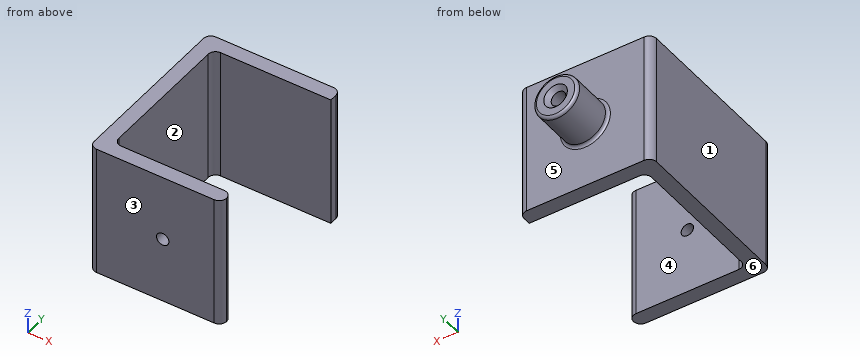
```python
from build123d import *

# Parameters (mm, degrees)
BOSS_EXTRUDE1_DEPTH         = 57.15
FILLET1_R                   = 6.35
FILLET2_R                   = 6.35
FILLET3_R                   = 6.35
F_1_2_13_TAPPED_HOLE1_D     = 10.71626
F_1_2_13_TAPPED_HOLE1_DEPTH = 12.7
SKETCH7_R                   = 19.05
BOSS_EXTRUDE2_DEPTH         = 38.1
SKETCH8_R                   = 8.382
CUT_EXTRUDE1_DEPTH          = 1.524
FILLET4_R                   = 2.54


with BuildPart() as part:
    # Sketch1 → Boss-Extrude1 (new, symmetric)
    with BuildSketch(Plane.XY):
        Polygon((0, 0), (0, 152.4), (114.3, 152.4), (114.3, 139.7), (12.7, 139.7), (12.7, 12.7), (114.3, 12.7), (114.3, 0), align=None)
    extrude(amount=BOSS_EXTRUDE1_DEPTH, both=True)

    # Fillet1
    fillet1_edges = [part.edges().sort_by_distance(p)[0] for p in [
        (12.7, 139.7, 0),
        (12.7, 12.7, 0),
    ]]
    fillet(fillet1_edges, radius=FILLET1_R)

    # Fillet2
    fillet2_edges = [part.edges().sort_by_distance(p)[0] for p in [
        (0, 0, 0),
        (0, 152.4, 0),
    ]]
    fillet(fillet2_edges, radius=FILLET2_R)

    # Fillet3
    fillet3_edges = [part.edges().sort_by_distance(p)[0] for p in [
        (114.3, 152.4, 0),
        (114.3, 12.7, 0),
        (114.3, 0, 0),
    ]]
    fillet(fillet3_edges, radius=FILLET3_R - 0.0001)  # a hair under: the kernel refuses the full size

    # 1/2-13 Tapped Hole1
    with Locations(Plane(origin=(0, 0, 0), x_dir=(-1, 0, 0), z_dir=(0, -1, 0))):
        with Locations((-63.5, 0)):
            Hole(F_1_2_13_TAPPED_HOLE1_D / 2, depth=F_1_2_13_TAPPED_HOLE1_DEPTH)

    # Sketch7 → Boss-Extrude2 (add)
    with BuildSketch(Plane(origin=(0, 152.4, 0), x_dir=(1, 0, 0), z_dir=(0, 1, 0))):
        with Locations((57.15, 0)):
            Circle(SKETCH7_R)
        with BuildLine():
            Line((58.42, 6.221703947), (58.42, 7.62))
            Line((58.42, 7.62), (55.88, 7.62))
            Line((55.88, 7.62), (55.88, 6.221703947))
            ThreePointArc((55.88, 6.221703947), (57.15, -6.35), (58.42, 6.221703947))
        make_face(mode=Mode.SUBTRACT)
    extrude(amount=BOSS_EXTRUDE2_DEPTH)

    # Sketch8 → Cut-Extrude1 (cut)
    with BuildSketch(Plane(origin=(0, 152.4, 0), x_dir=(1, 0, 0), z_dir=(0, 1, 0))):
        with Locations((57.15, 0)):
            Circle(SKETCH8_R)
    extrude(amount=CUT_EXTRUDE1_DEPTH, mode=Mode.SUBTRACT)

    # Fillet4
    fillet4_edges = [part.edges().sort_by_distance(p)[0] for p in [
        (38.1, 152.4, 0),
        (38.1, 190.5, 0),
    ]]
    fillet(fillet4_edges, radius=FILLET4_R)

    # Chamfer1: read off the stored shape, not the designer's step
    # Chamfer1 outline → Chamfer1 (revolve, cut)
    with BuildSketch(Plane(origin=(57.15, 0, 0), x_dir=(1, 0, 0), z_dir=(0, 0, 1))):
        Polygon((6.349999964, 190.5), (6.349999964, 186.689999964), (10.16, 190.5), align=None)
    revolve(axis=Axis((57.15, 0, 0), (0, 1, 0)), mode=Mode.SUBTRACT)


solid = part.part
```
Can you work these out from the model? Positions are in its coordinate system, mm. Face numbers are marked on the shaded views. A direction names the side the tool comes from. Coordinates: 2 decimals unless noted, no trailing zeros. Loops run counter-clockwise (first coordinate to the right, second up) from the corner with the lowest first, then second, coordinate; pieces in that order, holes last. Notation, with made-up numbers: (77.25, 75.25) - (128.25, 75.25) arc R25 ccw to (128.25, 89.25) - close; hole circle Ø6 at (76.25, 71.5). An arc over 180 degrees is marked (long way). Answer as CSV lines item,"result". Start each with the question number.
1) Suppose I cut it at C-C (y = 128). Please give me the cut outline in (x, z).
2) Thinking about a two-plate mould opening in Y: for the marked faces 1, 2 and 3, which applies, pulls with the +Y half, pulls with the -Y half, needs draft (parallel to the pull), parting line crosses it, or undercut?
3) I need wall thicknesses on line 1 (Y direction, x = 96, z = 24); line 2 (X direction, y = 178, z = 0); line 3 (Y direction, x = 50, z = 1.5). Which ranges of each line are inside material? Lowest first, please. Write a range as from..to.
4) Suppose I cut it at A-A (x = 81.5). Please give me the cut outline in (y, z).
5) For pin 1 (10 mm diameter, centred on x = 80, z = 6.5, fed in from +Y); pin 2 (1 mm diameter, centred on y = 155, z = 0.5, fed in from -X); pin 3 (8.5 mm diameter, centred on x = 58, z = 2.5, fed in from +Y), each with a flat end and sliding along its axis, tell me the tip position at first contact or that it passes through.
6) Which directions (+Z, -Z, +X, -X, +Y, -Y) give clear straight access to the entire face, cutting with the end or side of a thin tool? Please do the marked faces 4, 5 and 6.
Check result:
1,outline,"(0, -57.15) - (12.7, -57.15) - (12.7, 57.15) - (0, 57.15) - close"
2,face 1,"needs draft"
2,face 2,"undercut"
2,face 3,"pulls with the -Y half"
3,line 1,"y = 0..12.7, 139.7..152.4"
3,line 2,"x = 38.1..50.8, 63.5..76.2"
3,line 3,"y = 0..12.7, 139.7..152.4, 153.92..187.65"
4,outline,"(0, -57.15) - (12.7, -57.15) - (12.7, 57.15) - (0, 57.15) - close; (139.7, -57.15) - (152.4, -57.15) - (152.4, 57.15) - (139.7, 57.15) - close"
5,pin 1,"stops at y = 189.15"
5,pin 2,"stops at x = 38.07"
5,pin 3,"stops at y = 187.23"
6,face 4,"+Z, -Z, +X"
6,face 5,"+Y"
6,face 6,"-Z, +X, -X, +Y, -Y"
